Answer from the drawing. Dimensions are ordinates in mm from the lowest x, y and z of the part. A direction names the side the tool comes from. Round coordinates to 2 decimals unless told otherwise and drop trailing zeros. Loops run counter-clockwise (first coordinate to the right, second up) from the corner with the lowest first, then second, coordinate; pieces in that order, holes last. Notation, with made-up numbers: M -9,45.5 L 13,45.5 A25 cw 13,76.5 Z; hole C 85,81.25 d3. An arc over 180 degrees is marked long. Answer as a JSON object with one key per item and string values.
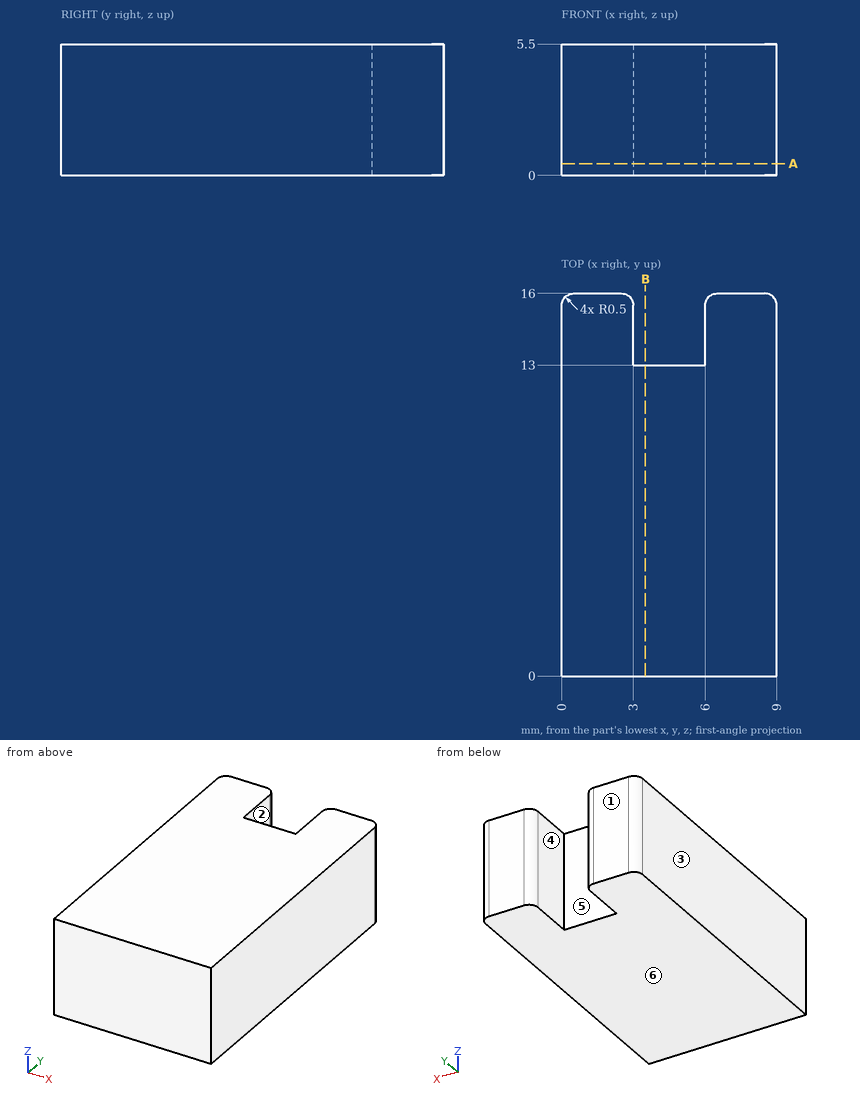
Item 1: Determine the mould class of the marked faces 3, 4, 5 and 6 for opening direction X: released by +X, released by -X, zero draft, split by the parting line, or undercut.
Values follow:
{"face 3": "released by -X", "face 4": "undercut", "face 5": "undercut", "face 6": "zero draft"}
Item 2: The part is cut by section B-B (x = 3.5). Give the vertices of the cut face in (y, z).
Values follow:
{"outline": "M 0,0 L 13,0 L 13,5.5 L 0,5.5 Z"}
Item 3: Which of the six approach directions +Z, -Z, +X, -X, +Y, -Y give full straight-line access (tool end or side, diameter ignored) to the marked faces 1 and 2?
Values follow:
{"face 1": "+Z, -Z, +X, -X, +Y", "face 2": "+Z, -Z, +Y"}
Item 4: The part is cut by section A-A (z = 0.5). Give the vertices of the cut face in (x, y), then the cut area to 3 significant figures.
Values follow:
{"outline": "M 0,0 L 9,0 L 9,15.5 A0.5 ccw 8.5,16 L 6.5,16 A0.5 ccw 6,15.5 L 6,13 L 3,13 L 3,15.5 A0.5 ccw 2.5,16 L 0.5,16 A0.5 ccw 0,15.5 Z", "area": "135 mm^2"}
Item 5: Straight lines are drawn through the part: line 1 (X direction, y = 15, z = 3.25); line 2 (Y direction, x = 4, z = 4.1); line 3 (Y direction, x = 8.75, z = 0.85). For each, find the intervals that lie inside material, in ascending order.
Values follow:
{"line 1": "0 to 3, 6 to 9", "line 2": "0 to 13", "line 3": "0 to 15.93"}
